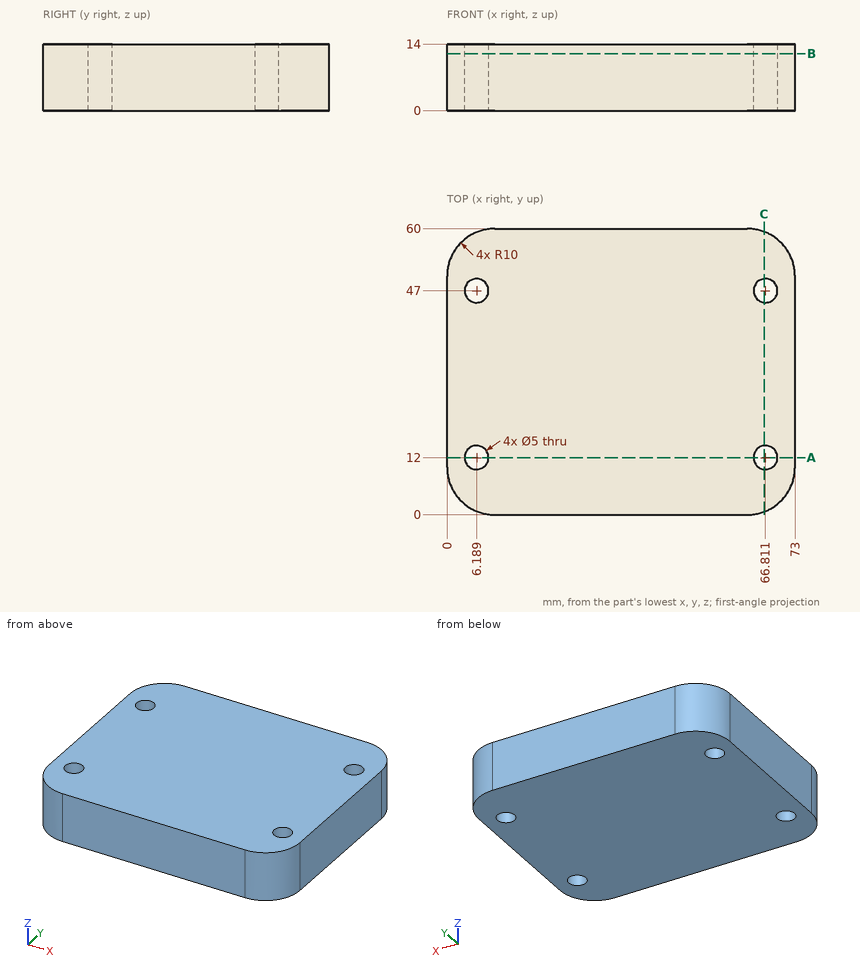
Can you work these out from the drawing? Everything is in mm from the part's minimum corner. Give positions to 0.01 mm unless a question says otherwise; leave off trailing zeros. Order: outer loops, then holes, each group sorted by start corner. A loop starts at its lowest first (then second) coordinate and runs counter-clockwise, first axis right, second up.
1. I need wall thicknesses on L1, parallel to X at y = 45.5, z = 10; L2, parallel to X at y = 14, z = 1.5; L3, parallel to X at y = 50.5, z = 7. Which ranges of each line are inside material? Lowest first, please.
2. Suppose I cut it at C-C (x = 66.5). List the corners of the cut face in (y, z) for me, plus the area to 3 significant figures.
3. Suppose I cut it at B-B (z = 12). List the corners of the cut face in (x, y) for me.
4. Suppose I cut it at A-A (y = 12). List the corners of the cut face in (x, z) for me.
Solved:
1. L1: x = 0 to 4.19, 8.19 to 64.81, 68.81 to 73
1. L2: x = 0 to 4.69, 7.69 to 65.31, 68.31 to 73
1. L3: x = 0.01 to 72.99
2. outline: (0.63, 0) - (9.52, 0) - (9.52, 14) - (0.63, 14) - close; (14.48, 0) - (44.52, 0) - (44.52, 14) - (14.48, 14) - close; (49.48, 0) - (59.37, 0) - (59.37, 14) - (49.48, 14) - close
2. area: 683 mm2
3. outline: (0, 10) arc R10 ccw to (10, 0) - (63, 0) arc R10 ccw to (73, 10) - (73, 50) arc R10 ccw to (63, 60) - (10, 60) arc R10 ccw to (0, 50) - close; hole circle Ø5 at (6.19, 12); hole circle Ø5 at (6.19, 47); hole circle Ø5 at (66.81, 12); hole circle Ø5 at (66.81, 47)
4. outline: (0, 0) - (3.69, 0) - (3.69, 14) - (0, 14) - close; (8.69, 0) - (64.31, 0) - (64.31, 14) - (8.69, 14) - close; (69.31, 0) - (73, 0) - (73, 14) - (69.31, 14) - close
